The model under review builds one solid part; all positions refer to its coordinate system, in mm. A direction names the side the tool comes from. Round coordinates to 2 decimals unless told otherwise and drop trailing zeros. Write each loop counter-clockwise with the first axis right and the second up, starting at its lowest first coordinate (ties: lowest second). Pieces come first, ordered by that corner, then holes. Notation, with made-up numbers: M 79.5,12.25 L 125.5,12.25 A21 cw 125.5,41.25 Z; hole C 27,82.25 d3. An arc over 180 degrees is marked long. One line per item, written item: value. Start each with the question number.
1) For P1, Ø15, axis at x = 16, y = -2.5, coming from the +Z side; P2, Ø1.6, axis at x = 70.5, y = 1, coming from the +Z side, all flat-tipped, find the tip position at first contact; note any pin that passes through.
2) Take a section at C-C, the plane y = 9.5. Write out the cut boundary in (x, z), and give its area (3 significant figures).
3) Take a section at D-D, the plane y = 0. Write out the cut boundary in (x, z), and give its area (3 significant figures).
4) Mouldability with a two-part tool opening along X and no side actions: class faces 4 (the face through (73, 0, 14)), 5 (the face through (-1, 0, 0)), 6 (the face through (-1, 0, 13)) as +X half, -X half, draft (parallel to the pull), parting line (faces both ways), or undercut.
5) Take a section at A-A, the plane x = -54. Write out the cut boundary in (y, z).
6) Take a section at B-B, the plane z = 21.5. Write out the cut boundary in (x, y).
7) Tool access review of faces 1 (the face through (-73, 0, 17)), 2 (the face through (70, 0, 28.5)), 3 (the face through (67.5, 0, 17)): name each direction out of +Z, -Z, +X, -X, +Y, -Y from which nothing blocks a thin tool from reaching the whole face with its end or side.
8) Wall thickness on probe 1 along X at (y, z) = (0, 17); probe 2 along Z at (x, y) = (-45, 0); probe 3 along Z at (x, y) = (-10, 9): over which ranges is each line inside the solid? List them lowest first.
Autodesk Inventor part; units mm, degrees
ref_plane "YZ Plane" through (0, 0, 0) normal (1, 0, 0) x (0, 1, 0)
ref_plane "XZ Plane" through (0, 0, 0) normal (0, 1, 0) x (-1, 0, 0)
ref_plane "XY Plane" through (0, 0, 0) normal (0, 0, 1) x (1, 0, 0)
sketch "Sketch1" plane through (0, 0, 0) normal (0, 0, 1) x (1, 0, 0)
  line L0 (73, -15) -> (-73, -15)
  line L1 (-73, -15) -> (-73, 15)
  line L2 (-73, 15) -> (73, 15)
  line L3 (73, 15) -> (73, -15)
  line L4 (73, -15) -> (-73, 15) construction
  line L5 (-73, -15) -> (73, 15) construction
  point P0 (0, 0)
  dimension "d0" = 146
  dimension "d1" = 30
extrude "Extrusion1" add sketch "Sketch1" along normal blind 13
sketch "Sketch2" plane through (0, 0, 13) normal (0, 0, 1) x (1, 0, 0)
  line L0 (-73, 15) -> (-73, -15)
  line L1 (-73, -15) -> (73, -15)
  line L2 (73, -15) -> (73, 15)
  line L3 (73, 15) -> (-73, 15)
  line L4 (-67.5, 15) -> (-67.5, -15)
  line L5 (67.5, 15) -> (67.5, -15)
  point P0 (0, 0)
  dimension "d4" = 5.5
  dimension "d5" = 5.5
extrude "Extrusion2" add sketch "Sketch2" along normal blind 22 contours L3 L4 L1 L0
extrude "Extrusion3" add sketch "Sketch2" along normal blind 15.5 contours L3 L2 L1 L5
sketch "Sketch3" plane through (-67.5, -15, 13) normal (1, 0, 0) x (0, 0, -1)
  line L0 (-22, 0) -> (0, 30)
  circle A0 centre (-11, 15) radius 4.5
  line L1 (-22, 0) -> (-22, 30)
  line L2 (-22, 15) -> (-12.5, 15)
  line L3 (-12.5, 15) -> (-8.5, 15)
  circle A1 centre (-8.5, 15) radius 4
  point P0 (13, 15)
  dimension "d10" = 9
  dimension "d21" = 9.5
  dimension "d22" = 4
extrude "Extrusion7" add sketch "Sketch3" along normal up to surface (135 mm away) contours A1 L3 L0 | L0 A0 A1 | A0 L0 A1 | L3 A1 A0 L0 | A1 L0 A0 picked at (-9.6413, 12.9367) picked at (-5.914, 15.6712) picked at (-8.2588, 18.8681)
thread "Thread2"
properties part number "linear trail"
Checked values:
1. P1: stops at z = 25.5
1. P2: stops at z = 28.5
2. outline: M -73,0 L 73,0 L 73,28.5 L 67.5,28.5 L 67.5,13 L -67.5,13 L -67.5,35 L -73,35 Z
2. area: 2,100 mm2
3. outline: M -73,0 L 73,0 L 73,28.5 L 67.5,28.5 L 67.5,25.5 L -67.5,25.5 L -67.5,35 L -73,35 Z; hole M -67.5,13 L 67.5,13 L 67.5,17.5 L -67.5,17.5 Z
3. area: 3,180 mm2
4. face 4: +X half
4. face 5: draft
4. face 6: undercut
5. outline: M -15,0 L 15,0 L 15,13 L -15,13 Z; C 0,21.5 d8
6. outline: M -73,-15 L -67.5,-15 L -67.5,-4 L 67.5,-4 L 67.5,-15 L 73,-15 L 73,15 L 67.5,15 L 67.5,4 L -67.5,4 L -67.5,15 L -73,15 Z
7. face 1: +Z, -Z, -X, +Y, -Y
7. face 2: +Z, +X, +Y, -Y
7. face 3: none
8. probe 1: x = -73 to -67.5, 67.5 to 73
8. probe 2: z = 0 to 13, 17.5 to 25.5
8. probe 3: z = 0 to 13
